```python
from build123d import *

# Parameters (mm, degrees)
F0_W      = 69.8630958796
F0_H      = 137.5265717506
F1_DEPTH  = 76.89179
F2_DEPTH  = 25.4
F3_DEPTH  = 25.4
F5_DEPTH  = 1676.4
F6_DEPTH  = 25.4
F8_DEPTH  = 25.4
F9_R      = 9.8377312504
F9_R_2    = 10.1939695419
F10_DEPTH = 2514.6


with BuildPart() as f1:
    # F0 (on Top) → F1 (new body)
    with BuildSketch(Plane.XY):
        with Locations((-34.9315479398, 0)):
            Rectangle(F0_W, F0_H)
        with Locations((34.9315479398, 0)):
            Rectangle(F0_W, F0_H)
    extrude(amount=-F1_DEPTH)

    # F2 (add): a face of the model
    f2_faces = [f1.faces().sort_by_distance(p)[0] for p in [
        (-69.8630958796, 0, -38.445895),
    ]]
    extrude(f2_faces, amount=-F2_DEPTH)

    # F3 (add): a face of the model
    f3_faces = [f1.faces().sort_by_distance(p)[0] for p in [
        (-69.8630958796, 0, -38.445895),
    ]]
    extrude(f3_faces, amount=F3_DEPTH)

    # F4 (on face) → F5 (cut)
    with BuildSketch(Plane.XZ.offset(68.7632858753)):
        with BuildLine():
            Line((29.3235648423, 0), (-56.6176436841, 0))
            ThreePointArc((-56.6176436841, 0), (-13.6470394209, -38.1281375917), (29.3235648423, 0))
        make_face()
    extrude(amount=-F5_DEPTH, mode=Mode.SUBTRACT)

    # F4 (on face) → F6 (join)
    with BuildSketch(Plane.XZ.offset(68.7632858753)):
        with BuildLine():
            Line((-56.6176436841, 0), (-69.2062154412, 0))
            ThreePointArc((-69.2062154412, 0), (-13.2839065045, -49.2343121992), (42.6384024322, 0))
            Line((42.6384024322, 0), (29.3235648423, 0))
            ThreePointArc((29.3235648423, 0), (-13.6470394209, -38.1281375917), (-56.6176436841, 0))
        make_face()
    extrude(amount=F6_DEPTH)

    # F7 (on face) → F8 (join)
    with BuildSketch(Plane(origin=(0, 68.7632858753, 0), x_dir=(-1, 0, 0), z_dir=(0, 1, 0))):
        with BuildLine():
            Line((-29.3235648423, 0), (-41.9121347368, 0))
            ThreePointArc((-41.9121347368, 0), (13.8891283423, -48.718451151), (69.6903914213, 0))
            Line((69.6903914213, 0), (56.6176436841, 0))
            ThreePointArc((56.6176436841, 0), (13.6470394209, -38.1281375917), (-29.3235648423, 0))
        make_face()
    extrude(amount=F8_DEPTH)

    # F9 (on face) → F10 (cut)
    with BuildSketch(Plane.XY):
        with Locations((-76.6867026687, 0)):
            Circle(F9_R)
        with Locations((49.7599355876, 0)):
            Circle(F9_R_2)
    extrude(amount=-F10_DEPTH, mode=Mode.SUBTRACT)


solid = f1.part
```
The listing builds one solid part. Answer for the finished solid, in the listing's coordinates (mm). A direction names the side the tool comes from. Coordinates: 2 decimals unless noted, no trailing zeros. Write each loop counter-clockwise with the first axis right and the second up, starting at its lowest first coordinate (ties: lowest second). Pieces come first, ordered by that corner, then holes. Notation, with made-up numbers: (-32, 75.5) - (-8, 75.5) arc R26 cw to (-8, 93.5) - close; hole circle Ø10 at (33, -20.75). An arc over 180 degrees is marked (long way). One line per item, written item: value.
1) Find section D-D (y = -32.5). Give the vertices of the cut face in (x, z).
Geometry check:
outline: (-95.26, -76.89) - (69.86, -76.89) - (69.86, 0) - (29.32, 0) arc R43.28 cw to (-56.62, 0) - (-95.26, 0) - close
2) For a pull along X with two mould halves and no side action, classify faces 4 (the flat face through (-95.263, -1, -38)), 5 (the flat face through (-12, -68.763, -55)), 6 (the cylindrical face through (-14.53, -1.32, -38.12)) as pulls with the +X half, pulls with the -X half, needs draft (parallel to the pull), parting line crosses it, or undercut.
Geometry check:
face 4: pulls with the -X half
face 5: needs draft
face 6: undercut
3) Find section C-C (x = 47.5). Give the vertices of the cut face in (y, z), and give its area (3 significant figures).
Geometry check:
outline: (-68.76, -76.89) - (-9.94, -76.89) - (-9.94, 0) - (-68.76, 0) - close; (9.94, -76.89) - (68.76, -76.89) - (68.76, 0) - (9.94, 0) - close
area: 9,050 mm2
4) Find section A-A (z = -18). Give the vertices of the cut face in (x, y).
Geometry check:
outline: (-95.26, -68.76) - (-63.74, -68.76) - (-63.74, -94.16) - (-50.21, -94.16) - (-50.21, 94.16) - (-64.05, 94.16) - (-64.05, 68.76) - (-95.26, 68.76) - close; (22.92, -94.16) - (37.18, -94.16) - (37.18, -68.76) - (69.86, -68.76) - (69.86, 68.76) - (36.27, 68.76) - (36.27, 94.16) - (22.92, 94.16) - close; hole circle Ø19.68 at (-76.69, 0); hole circle Ø20.39 at (49.76, 0)
5) A tool of negligible diameter and unlimited length cuts with its end or side. For faces 1 (the cylindrical face through (-14.423, -81.285, -49.223)), 2 (the cylindrical face through (-12.757, 81.285, -48.707)), 3 (the cylindrical face through (59.18, -3.9, -37.91)), from which of +Z, -Z, +X, -X, +Y, -Y can it reach the whole face along a straight path? Write none if from no direction.
Geometry check:
face 1: -Z, -Y
face 2: -Z, +Y
face 3: +Z, -Z
6) Consider line 1 along Y through (x, z) = (-21.5, -48.5); line 2 along X through (y, z) = (-84, -20.5); line 3 along X through (y, z) = (66, -29.5). Determine where each line is inside the solid, lowest interval first. Write a range as from..to.
Geometry check:
line 1: y = -94.16..68.76
line 2: x = -62.42..-48.5, 21.21..35.85
line 3: x = -95.26..-39.58, 12.28..69.86
7) Find section B-B (y = 0). Give the vertices of the cut face in (x, z), and give its area (3 significant figures).
Geometry check:
outline: (-95.26, -76.89) - (-86.52, -76.89) - (-86.52, 0) - (-95.26, 0) - close; (-66.85, -76.89) - (39.57, -76.89) - (39.57, 0) - (29.32, 0) arc R43.28 cw to (-56.62, 0) - (-66.85, 0) - close; (59.95, -76.89) - (69.86, -76.89) - (69.86, 0) - (59.95, 0) - close
area: 7,120 mm2
8) Each of these flat-tipped pins is pushed along its axis until it touches: pin 1 Ø23 at (x, z) = (-42, -49) entering from +Y; pin 2 Ø6 at (x, y) = (-39, 75) entering from -Z; pin 3 Ø2 at (x, y) = (-35, 71.5) entering from -Z; pin 4 Ø12 at (x, y) = (-23.5, -53) entering from +Z. Where does it stop, or does it pass through?
Geometry check:
pin 1: stops at y = 94.16
pin 2: stops at z = -44.2
pin 3: stops at z = -45.01
pin 4: stops at z = -35.12
